```python
from build123d import *

# Parameters (mm, degrees)
SKETCH_1_W             = 140
SKETCH_1_H             = 200
SKETCH_1_R             = 1.5
EXTRUDE_1_DEPTH        = 4
SKETCH_2_W             = 20
SKETCH_2_H             = 20
EXTRUDE_2_DEPTH        = 4
FILLET_1_R             = 3
FILLET_1_OF_MIRROR_1_R = 3
SKETCH_3_W             = 8
SKETCH_3_H             = 30
SKETCH_3_R             = 1.75
EXTRUDE_3_DEPTH        = 4
FILLET_2_R             = 3
FILLET_2_OF_MIRROR_2_R = 3
FILLET_3_R             = 5
EXTRUDE_4_DEPTH        = 4
SKETCH_5_R             = 1.75
CUT_EXTRUDE_1_DEPTH    = 10
SKETCH_6_W             = 30
SKETCH_6_H             = 60
CUT_EXTRUDE_2_DEPTH    = 10
SKETCH_7_R             = 2.112337694
SKETCH_7_R_2           = 2
CUT_EXTRUDE_3_DEPTH    = 10


with BuildPart() as part:
    # 草图1 → 凸台-拉伸1 (new body)
    with BuildSketch(Plane.XY):
        Rectangle(SKETCH_1_W, SKETCH_1_H)
        with Locations((-65, 40)):
            Circle(SKETCH_1_R, mode=Mode.SUBTRACT)
        with Locations(Location((-65, -40, 0), (0, 0, 180))):
            Circle(SKETCH_1_R, mode=Mode.SUBTRACT)
        with Locations((65, -40)):
            Circle(SKETCH_1_R, mode=Mode.SUBTRACT)
        with Locations(Location((65, 40, 0), (0, 0, 180))):
            Circle(SKETCH_1_R, mode=Mode.SUBTRACT)
    extrude(amount=EXTRUDE_1_DEPTH)

    # 草图2 → 凸台-拉伸2 (add)
    with BuildSketch(Plane.XY.offset(4)):
        with Locations((80, 90)):
            Rectangle(SKETCH_2_W, SKETCH_2_H)
    extrude_2 = extrude(amount=-EXTRUDE_2_DEPTH)

    # 圆角1
    fillet_1_edges = [part.edges().sort_by_distance(p)[0] for p in [
        (90, 100, 2),
        (90, 80, 2),
    ]]
    fillet(fillet_1_edges, radius=FILLET_1_R)

    # 镜向1: 凸台-拉伸2 across plane
    add(extrude_2.mirror(Plane(origin=(0, 0, 0), x_dir=(0, 0, 1), z_dir=(1, 0, 0))))

    # 圆角1 of 镜向1
    fillet_1_of_mirror_1_edges = [part.edges().sort_by_distance(p)[0] for p in [
        (-90, 100, 2),
        (-90, 80, 2),
    ]]
    fillet(fillet_1_of_mirror_1_edges, radius=FILLET_1_OF_MIRROR_1_R)

    # 草图3 → 凸台-拉伸3 (add)
    with BuildSketch(Plane.XY.offset(4)):
        with Locations((-66, 115)):
            Rectangle(SKETCH_3_W, SKETCH_3_H)
        with Locations((-66, 126)):
            Circle(SKETCH_3_R, mode=Mode.SUBTRACT)
    extrude_3 = extrude(amount=-EXTRUDE_3_DEPTH)

    # 圆角2
    fillet_2_edges = [part.edges().sort_by_distance(p)[0] for p in [
        (-70, 100, 2),
        (-62, 100, 2),
    ]]
    fillet(fillet_2_edges, radius=FILLET_2_R)

    # 镜向2: 凸台-拉伸3 across plane
    add(extrude_3.mirror(Plane(origin=(0, 0, 0), x_dir=(0, 0, 1), z_dir=(1, 0, 0))))

    # 圆角2 of 镜向2
    fillet_2_of_mirror_2_edges = [part.edges().sort_by_distance(p)[0] for p in [
        (70, 100, 2),
        (62, 100, 2),
    ]]
    fillet(fillet_2_of_mirror_2_edges, radius=FILLET_2_OF_MIRROR_2_R)

    # 圆角3
    fillet_3_edges = [part.edges().sort_by_distance(p)[0] for p in [
        (-70, -100, 2),
        (70, -100, 2),
    ]]
    fillet(fillet_3_edges, radius=FILLET_3_R)

    # 草图4 → 凸台-拉伸4 (add)
    with BuildSketch(Plane(origin=(0, 0, 0), x_dir=(-1, 0, 0), z_dir=(0, 0, -1))):
        with BuildLine():
            add(Edge.make_bspline(
                [(-33.786379938, 100), (-33.384771108, 111.24314249), (-38.944167614, 121.897129031), (-48.25387443, 128.002822688)],
                knots=[0, 0, 0, 0, 0.66194058, 0.66194058, 0.66194058, 0.66194058], degree=3))
            Line((-33.786379938, 100), (0, 100))
            ThreePointArc((0, 100), (-9.331566745, 102.310402433), (-16.507166038, 108.707813791))
            ThreePointArc((-16.507166038, 108.707813791), (-29.663945789, 122.555538901), (-46.506293223, 131.566403293))
            ThreePointArc((-46.506293223, 131.566403293), (-48.952735362, 130.555841868), (-48.25387443, 128.002822688))
        make_face()
        with BuildLine():
            ThreePointArc((16.507166038, 108.707813791), (9.331566745, 102.310402433), (0, 100))
            Line((0, 100), (33.786379938, 100))
            add(Edge.make_bspline(
                [(33.786379938, 100), (33.384771108, 111.24314249), (38.944167614, 121.897129031), (48.25387443, 128.002822688)],
                knots=[0, 0, 0, 0, 0.66194058, 0.66194058, 0.66194058, 0.66194058], degree=3))
            ThreePointArc((48.25387443, 128.002822688), (48.952735362, 130.555841868), (46.506293223, 131.566403293))
            ThreePointArc((46.506293223, 131.566403293), (29.663945789, 122.555538901), (16.507166038, 108.707813791))
        make_face()
    extrude(amount=-EXTRUDE_4_DEPTH)

    # 草图5 → 切除-拉伸1 (cut)
    with BuildSketch(Plane(origin=(0, 0, 0), x_dir=(-1, 0, 0), z_dir=(0, 0, -1))):
        with BuildLine():
            Line((-70, 80), (-70, 60))
            Line((-70, 60), (70, 60))
            Line((70, 60), (70, 80))
            Line((70, 80), (87, 80))
            ThreePointArc((87, 80), (89.121320344, 80.878679656), (90, 83))
            Line((90, 83), (90, 97))
            ThreePointArc((90, 97), (89.121320344, 99.121320344), (87, 100))
            Line((87, 100), (73, 100))
            ThreePointArc((73, 100), (70.878679656, 100.878679656), (70, 103))
            Line((70, 103), (70, 130))
            Line((70, 130), (62, 130))
            Line((62, 130), (62, 103))
            ThreePointArc((62, 103), (61.121320344, 100.878679656), (59, 100))
            Line((59, 100), (33.786379938, 100))
            add(Edge.make_bspline(
                [(33.786379938, 100), (33.384771108, 111.24314249), (38.944167614, 121.897129031), (48.25387443, 128.002822688)],
                knots=[0, 0, 0, 0, 0.66194058, 0.66194058, 0.66194058, 0.66194058], degree=3))
            ThreePointArc((48.25387443, 128.002822688), (48.952735362, 130.555841868), (46.506293223, 131.566403293))
            ThreePointArc((46.506293223, 131.566403293), (29.663945789, 122.555538901), (16.507166038, 108.707813791))
            ThreePointArc((16.507166038, 108.707813791), (0, 100), (-16.507166038, 108.707813791))
            ThreePointArc((-16.507166038, 108.707813791), (-29.663945789, 122.555538901), (-46.506293223, 131.566403293))
            ThreePointArc((-46.506293223, 131.566403293), (-48.952735362, 130.555841868), (-48.25387443, 128.002822688))
            add(Edge.make_bspline(
                [(-48.25387443, 128.002822688), (-38.944167614, 121.897129031), (-33.384771108, 111.24314249), (-33.786379938, 100)],
                knots=[0, 0, 0, 0, 0.66194058, 0.66194058, 0.66194058, 0.66194058], degree=3))
            Line((-33.786379938, 100), (-59, 100))
            ThreePointArc((-59, 100), (-61.121320344, 100.878679656), (-62, 103))
            Line((-62, 103), (-62, 130))
            Line((-62, 130), (-70, 130))
            Line((-70, 130), (-70, 103))
            ThreePointArc((-70, 103), (-70.878679656, 100.878679656), (-73, 100))
            Line((-73, 100), (-87, 100))
            ThreePointArc((-87, 100), (-89.121320344, 99.121320344), (-90, 97))
            Line((-90, 97), (-90, 83))
            ThreePointArc((-90, 83), (-89.121320344, 80.878679656), (-87, 80))
            Line((-87, 80), (-70, 80))
        make_face()
        with Locations((-66, 126)):
            Circle(SKETCH_5_R, mode=Mode.SUBTRACT)
        with Locations((66, 126)):
            Circle(SKETCH_5_R, mode=Mode.SUBTRACT)
    extrude(amount=-CUT_EXTRUDE_1_DEPTH, mode=Mode.SUBTRACT)

    # 草图6 → 切除-拉伸2 (cut)
    with BuildSketch(Plane(origin=(0, 0, 0), x_dir=(-1, 0, 0), z_dir=(0, 0, -1))):
        with Locations((0, 30)):
            Rectangle(SKETCH_6_W, SKETCH_6_H)
    extrude(amount=-CUT_EXTRUDE_2_DEPTH, mode=Mode.SUBTRACT)

    # 草图7 → 切除-拉伸3 (cut)
    with BuildSketch(Plane.XY.offset(4)):
        with Locations((56.25, 51.25)):
            Circle(SKETCH_7_R)
        with Locations((56.25, -23.25)):
            Circle(SKETCH_7_R)
        with Locations((21.75, 51.25)):
            Circle(SKETCH_7_R)
        with Locations((21.75, -23.25)):
            Circle(SKETCH_7_R)
        with Locations((43.610044526, -35)):
            Circle(SKETCH_7_R_2)
        with Locations((50.610044526, -82)):
            Circle(SKETCH_7_R_2)
        with Locations((-31.889955474, -35)):
            Circle(SKETCH_7_R_2)
        with Locations((-31.889955474, -82)):
            Circle(SKETCH_7_R_2)
        with Locations((-24, 47)):
            Circle(SKETCH_7_R_2)
        with Locations((-57, 47)):
            Circle(SKETCH_7_R_2)
        with Locations((-24, -14)):
            Circle(SKETCH_7_R_2)
        with Locations((-57, -14)):
            Circle(SKETCH_7_R_2)
    extrude(amount=-CUT_EXTRUDE_3_DEPTH, mode=Mode.SUBTRACT)


solid = part.part
```
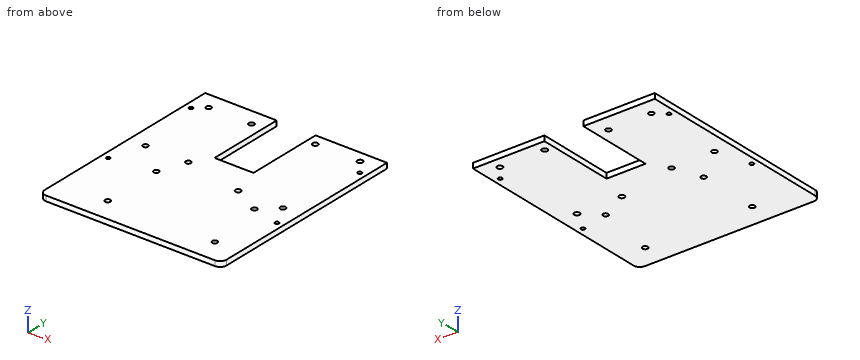
Read the model definition and answer for the solid it produces. Units are mm, in the model's axes. Give positions to 0.01 mm unless a question says otherwise; leave off trailing zeros. Order: outer loops, then holes, each group sorted by start corner. A loop starts at its lowest first (then second) coordinate and runs counter-clockwise, first axis right, second up.
(1) Straight lines are drawn through the part: L1, parallel to Y at x = -65, z = 1.9; L2, parallel to X at y = 51, z = 1; L3, parallel to X at y = 40.5, z = 2.75. For each, find the intervals that lie inside material, in ascending order.
(2) Find section A-A (y = 15). Give the vertices of the cut face in (x, z).
(3) Find section D-D (x = 21.75). Give the vertices of the cut face in (y, z).
(4) Find section B-B (y = -82). Give the vertices of the cut face in (x, z).
(5) Find section C-C (z = 1.95). Give the number of separate pieces and of enclosed holes in the cut face, plus the area to 3 significant figures.
Result sheet:
1. L1: y = -100 to -41.5, -38.5 to 38.5, 41.5 to 60
1. L2: x = -70 to -15, 15 to 19.65, 23.85 to 54.15, 58.35 to 70
1. L3: x = -70 to -66.41, -63.59 to -15, 15 to 63.59, 66.41 to 70
2. outline: (-70, 0) - (-15, 0) - (-15, 4) - (-70, 4) - close; (15, 0) - (70, 0) - (70, 4) - (15, 4) - close
3. outline: (-100, 0) - (-25.36, 0) - (-25.36, 4) - (-100, 4) - close; (-21.14, 0) - (49.14, 0) - (49.14, 4) - (-21.14, 4) - close; (53.36, 0) - (60, 0) - (60, 4) - (53.36, 4) - close
4. outline: (-70, 0) - (-33.89, 0) - (-33.89, 4) - (-70, 4) - close; (-29.89, 0) - (48.61, 0) - (48.61, 4) - (-29.89, 4) - close; (52.61, 0) - (70, 0) - (70, 4) - (52.61, 4) - close
5. separate pieces: 1
5. enclosed holes: 16
5. area: 20,400 mm2
